```python
from build123d import *

# Parameters (mm, degrees)
BOSS_EXTRUDE1_DEPTH                             = 6.35
CSK_FOR_M6_FLAT_HEAD_MACHINE_SCREW1_D           = 6.6
CSK_FOR_M6_FLAT_HEAD_MACHINE_SCREW1_CSINK_D     = 12.6
CSK_FOR_M6_FLAT_HEAD_MACHINE_SCREW1_CSINK_ANGLE = 90
CSK_FOR_M6_FLAT_HEAD_MACHINE_SCREW2_D           = 6.6
CSK_FOR_M6_FLAT_HEAD_MACHINE_SCREW2_CSINK_D     = 12.6
CSK_FOR_M6_FLAT_HEAD_MACHINE_SCREW2_CSINK_ANGLE = 90


with BuildPart() as part:
    # Sketch2 → Boss-Extrude1 (new body)
    # profile 1 of 3: a face of its own
    with BuildSketch(Plane(origin=(0, 0, 0), x_dir=(0, 0, -1), z_dir=(1, 0, 0))):
        Polygon((-134.915615546, 101.6), (-134.915615546, 0), (-46.015615546, 0), (-46.015615546, 50.8), (-46.015615546, 101.6), align=None)
        with BuildLine():
            Line((-103.431783211, 79.375), (-103.431783211, 50.8))
            Line((-103.431783211, 50.8), (-103.431783211, 22.225))
            ThreePointArc((-103.431783211, 22.225), (-109.515615546, 16.141167665), (-115.599447882, 22.225))
            Line((-115.599447882, 22.225), (-115.599447882, 79.375))
            ThreePointArc((-115.599447882, 79.375), (-109.515615546, 85.458832335), (-103.431783211, 79.375))
        make_face(mode=Mode.SUBTRACT)
    # profile 2 of 3: a face of its own
    with BuildSketch(Plane(origin=(0, 0, 0), x_dir=(0, 0, -1), z_dir=(1, 0, 0))):
        Polygon((42.884384454, 203.2), (-134.915615546, 101.6), (-46.015615546, 101.6), (42.884384454, 101.6), align=None)
    # profile 3 of 3: a face of its own
    with BuildSketch(Plane(origin=(0, 0, 0), x_dir=(0, 0, -1), z_dir=(1, 0, 0))):
        Polygon((-46.015615546, 50.8), (-46.015615546, 0), (42.884384454, 0), (42.884384454, 101.6), (-46.015615546, 101.6), align=None)
        with BuildLine():
            Line((11.400552118, 22.225), (11.400552118, 50.8))
            Line((11.400552118, 50.8), (11.400552118, 79.375))
            ThreePointArc((11.400552118, 79.375), (17.484384454, 85.458832335), (23.568216789, 79.375))
            Line((23.568216789, 79.375), (23.568216789, 22.225))
            ThreePointArc((23.568216789, 22.225), (17.484384454, 16.141167665), (11.400552118, 22.225))
        make_face(mode=Mode.SUBTRACT)
    extrude(amount=BOSS_EXTRUDE1_DEPTH)

    # CSK for M6 Flat Head Machine Screw1 (through all)
    with Locations(Plane(origin=(6.35, 0, 0), x_dir=(0, 0, -1), z_dir=(1, 0, 0))):
        with Locations((-81.575615546, 15.24), (-81.575615546, 88.9), (-61.255615546, 88.9), (-61.255615546, 15.24)):
            CounterSinkHole(CSK_FOR_M6_FLAT_HEAD_MACHINE_SCREW1_D / 2, CSK_FOR_M6_FLAT_HEAD_MACHINE_SCREW1_CSINK_D / 2, counter_sink_angle=CSK_FOR_M6_FLAT_HEAD_MACHINE_SCREW1_CSINK_ANGLE)

    # CSK for M6 Flat Head Machine Screw2 (through all)
    with Locations(Plane(origin=(6.35, 0, 0), x_dir=(0, 0, -1), z_dir=(1, 0, 0))):
        with Locations((-65.065615546, 114.3), (-33.315615546, 127), (-1.565615546, 127), (-1.565615546, 152.4)):
            CounterSinkHole(CSK_FOR_M6_FLAT_HEAD_MACHINE_SCREW2_D / 2, CSK_FOR_M6_FLAT_HEAD_MACHINE_SCREW2_CSINK_D / 2, counter_sink_angle=CSK_FOR_M6_FLAT_HEAD_MACHINE_SCREW2_CSINK_ANGLE)


solid = part.part
```
Work out the finished part from the listing and answer in its coordinate system (mm). A direction names the side the tool comes from. Round coordinates to 2 decimals unless told otherwise and drop trailing zeros. Write each loop counter-clockwise with the first axis right and the second up, starting at its lowest first coordinate (ties: lowest second). Pieces come first, ordered by that corner, then holes.
1) A cutting plane is placed at C-C on y = 114.3. Determine the outline of the cut face in (x, z), and give its area (3 significant figures).
2) A cutting plane is placed at D-D on z = 106. Determine the outline of the cut face in (x, y), and give its area (3 significant figures).
3) Which of the six approach directions +Z, -Z, +X, -X, +Y, -Y give full straight-line access (tool end or side, diameter ignored) to faces 4 (the face through (6.35, 80, 28)), 5 (the face through (3, 50, 115.599))?
4) A cutting plane is placed at B-B on y = 88.9. Determine the outline of the cut face in (x, z), and give its area (3 significant figures).
5) Flat-ended cylindrical pins translate along their axes: P1, Ø2, axis at x = 1.5, z = 43.5, coming from the +Y side; P2, Ø10.5, axis at y = 15.24, z = 81.58, coming from the +X side; P3, Ø1, axis at x = 4, z = -15, coming from the +Y side. Find the tip coordinate at first contact, or state that the pin passes through.
6) Determine the mould class of faces 1 (the face through (3.13, 153.11, 44.77)), 2 (the face through (0, 80, 28)), 3 (the face through (3.496, 115.335, 68.352)) for opening direction Y: pulls with the +Y half, pulls with the -Y half, needs draft (parallel to the pull), parting line crosses it, or undercut.
7) Consider probe 1 along Z at (x, y) = (3, 57); probe 2 along Z at (x, y) = (1.25, 15.24); probe 3 along Y at (x, z) = (5.75, 0.5). Determine where each line is inside the solid, lowest interval first.
8) A cutting plane is placed at A-A on x = 1.5. Give the number of separate pieces and of enclosed holes in the cut face, and give its area (3 significant figures).
Entries:
1. outline: (0, -42.88) - (6.35, -42.88) - (6.35, 58.77) - (3.35, 61.77) - (0, 61.77) - close; (0, 68.37) - (3.35, 68.37) - (6.35, 71.37) - (6.35, 112.69) - (0, 112.69) - close
1. area: 937 mm2
2. outline: (0, 0) - (6.35, 0) - (6.35, 17.26) - (0, 17.26) - close; (0, 84.34) - (6.35, 84.34) - (6.35, 118.12) - (0, 118.12) - close
2. area: 324 mm2
3. face 4: +Z, -Z, +X, +Y, -Y
3. face 5: +X, -X
4. outline: (0, -42.88) - (6.35, -42.88) - (6.35, 54.96) - (3.35, 57.96) - (0, 57.96) - close; (0, 64.56) - (3.35, 64.56) - (6.35, 67.56) - (6.35, 75.28) - (3.35, 78.28) - (0, 78.28) - close; (0, 84.88) - (3.35, 84.88) - (6.35, 87.88) - (6.35, 134.92) - (0, 134.92) - close
4. area: 1,030 mm2
5. P1: stops at y = 154.41
5. P2: stops at x = 5.3
5. P3: stops at y = 187.55
6. face 1: pulls with the +Y half
6. face 2: needs draft
6. face 3: undercut
7. probe 1: z = -42.88 to -23.57, -11.4 to 103.43, 115.6 to 134.92
7. probe 2: z = -42.88 to 57.96, 64.56 to 78.28, 84.88 to 134.92
7. probe 3: y = 0 to 121.4, 132.6 to 146.8, 158 to 178.41
8. separate pieces: 1
8. enclosed holes: 10
8. area: 25,200 mm2
